CAD build for the part. Positions are in the model's coordinates, mm. Face numbers are marked on the shaded views. A direction names the side the tool comes from. Give positions to 0.01 mm unless a question says otherwise; leave off trailing zeros. Order: outer loops, then holes, each group sorted by start corner. A loop starts at its lowest first (then second) coordinate and runs counter-clockwise, first axis right, second up.
Item 1: Band-saw the part on C-C on y = 9.5. Give the cut face in (x, z), plus the area to 3 significant figures.
Item 2: Flat gauge pins, fed straight in: P1, Ø8, axis at y = 14, z = 35.5, coming from the +X side; P2, Ø3, axis at y = -3, z = 15, coming from the -X side; P3, Ø2, axis at y = -17.5, z = 50, coming from the -X side. Where does each tip first touch, or does it go through?
Item 3: Band-saw the part on A-A on x = 0. Give the cut face in (y, z), plus the area to 3 significant figures.
Item 4: Two-plate mould, pull along Z, no slides. Class the marked faces 1, 2 and 3: released by +Z, released by -Z, zero draft, split by the parting line, or undercut.
Item 5: Wall check: L1, parallel to Z at x = 0, y = -10; L2, parallel to Z at x = 0, y = 0; L3, parallel to X at y = 15.5, z = 2. Give the ranges that are in metal, low to high.
Item 6: Band-saw the part on D-D on y = -0.5. Give the cut face in (x, z), plus the area to 3 significant figures.
Item 7: Which spindle directions (+Z, -Z, +X, -X, +Y, -Y) get a long thin tool onto all of the face, cutting with end or side? Do the marked faces 4 and 5. Say none if no direction does.
Item 8: Band-saw the part on B-B on z = 0. Give the cut face in (x, y), plus the area to 3 significant figures.
```python
from build123d import *

# Parameters (mm, degrees)
F0_R         = 68.25
F0_R_2       = 12.5
F1_DEPTH     = 25.4
F2_W         = 8
F2_H         = 15.8
F3_DEPTH     = 50.801
F4_R         = 78.15
F4_R_2       = 20
F5_DEPTH     = 7.5
F6_S5_R      = 68.25
F6_T6_DEPTH  = 112
F6_S11_R     = 68.25
F6_T12_DEPTH = 112


# Not quite as in the source:
# - a fillet or chamfer that OpenCascade refuses, or shapes differently, is made with other operations: its cross-section is extruded or revolved along the edge and cut away or added


with BuildPart() as f1:
    # F0 (on Front) → F1 (new body, symmetric)
    with BuildSketch(Plane.XZ):
        Circle(F0_R)
        Circle(F0_R_2, mode=Mode.SUBTRACT)
    extrude(amount=F1_DEPTH, both=True)

    # F2 (on face) → F3 (cut, through all)
    with BuildSketch(Plane.XZ.offset(25.4)):
        with Locations((0, 7.9)):
            Rectangle(F2_W, F2_H)
    extrude(amount=-F3_DEPTH, mode=Mode.SUBTRACT)

    # F4 (on Front) → F5 (join, symmetric)
    with BuildSketch(Plane.XZ):
        Circle(F4_R)
        Circle(F4_R_2, mode=Mode.SUBTRACT)
    extrude(amount=F5_DEPTH, both=True)

    # F6: chamfer of 10 x 3.6397023427 on 2 edges, made by hand


with BuildPart() as f6_tool2:
    # F6_s3 → F6_t4 (revolve)
    with BuildSketch(Plane.XY):
        Polygon((78.15, -3.8602976573), (68.15, -7.5), (78.15, -7.5), align=None)
    revolve(axis=Axis((0, -7.5, 0), (0, -1, 0)))

    # F6_s5 → F6_t6 (cut, symmetric)
    with BuildSketch(Plane.XZ.offset(5.7)):
        Circle(F6_S5_R)
    extrude(amount=F6_T6_DEPTH, both=True, mode=Mode.SUBTRACT)


with BuildPart() as f1_1:
    add(f1.part)

    # F6_t1: cut F6_tool2
    add(f6_tool2.part, mode=Mode.SUBTRACT)


with BuildPart() as f6_tool8:
    # F6_s9 → F6_t10 (revolve)
    with BuildSketch(Plane.XY):
        Polygon((68.15, 7.5), (78.15, 3.8602976573), (78.15, 7.5), align=None)
    revolve(axis=Axis((0, 7.5, 0), (0, -1, 0)))

    # F6_s11 → F6_t12 (cut, symmetric)
    with BuildSketch(Plane.XZ.offset(-5.7)):
        Circle(F6_S11_R)
    extrude(amount=F6_T12_DEPTH, both=True, mode=Mode.SUBTRACT)


with BuildPart() as f1_2:
    add(f1_1.part)

    # F6_t7: cut F6_tool8
    add(f6_tool8.part, mode=Mode.SUBTRACT)


solid = f1_2.part
```
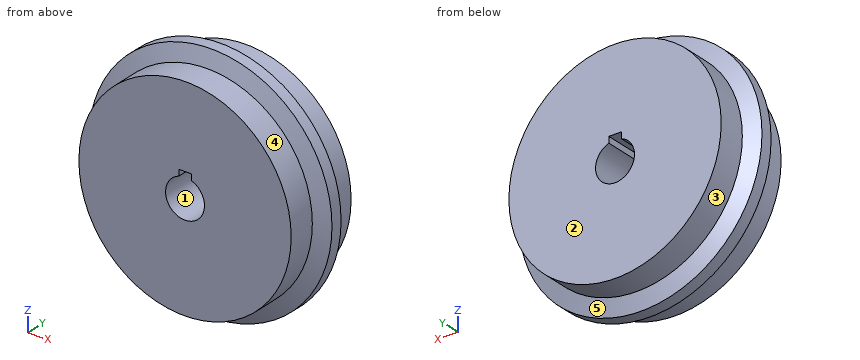
The answers:
1. outline: circle Ø136.5 at (0, 0); hole (-4, 11.84) arc R12.5 ccw (long way) to (4, 11.84) - (4, 15.8) - (-4, 15.8) - close
1. area: 14,100 mm2
2. P1: stops at x = 60.55
2. P2: stops at x = -76.98
2. P3: stops at x = -47.51
3. outline: (-25.4, -68.25) - (-7.46, -68.25) - (-3.86, -78.15) - (3.86, -78.15) - (7.46, -68.25) - (25.4, -68.25) - (25.4, -12.5) - (-25.4, -12.5) - close; (-25.4, 15.8) - (25.4, 15.8) - (25.4, 68.25) - (7.46, 68.25) - (3.86, 78.15) - (-3.86, 78.15) - (-7.46, 68.25) - (-25.4, 68.25) - close
3. area: 5,720 mm2
4. face 1: undercut
4. face 2: zero draft
4. face 3: split by the parting line
5. L1: z = -68.25 to -12.5, 15.8 to 68.25
5. L2: z = -78.15 to -12.5, 15.8 to 78.15
5. L3: x = -68.22 to -12.34, 12.34 to 68.22
6. outline: circle Ø156.3 at (0, 0); hole (-4, 11.84) arc R12.5 ccw (long way) to (4, 11.84) - (4, 15.8) - (-4, 15.8) - close
6. area: 18,700 mm2
7. face 4: -Y
7. face 5: +Y
8. outline: (-78.15, -3.86) - (-68.25, -7.46) - (-68.25, -25.4) - (-12.5, -25.4) - (-12.5, 25.4) - (-68.25, 25.4) - (-68.25, 7.46) - (-78.15, 3.86) - close; (12.5, -25.4) - (68.25, -25.4) - (68.25, -7.46) - (78.15, -3.86) - (78.15, 3.86) - (68.25, 7.46) - (68.25, 25.4) - (12.5, 25.4) - close
8. area: 5,890 mm2
